Drawing for the job (mm, zero at the part's lowest x, y, z). A direction names the side the tool comes from. Give positions to 0.01 mm unless a question says otherwise; leave off trailing zeros. Order: outer loops, then holes, each group sorted by start corner. A loop starts at its lowest first (then second) coordinate and runs counter-clockwise, first axis right, second up. Notation, with made-up numbers: (35, 0.25) - (54, 0.25) arc R13 cw to (54, 9.25) - close; hole circle Ø1 at (85, 57.5). An arc over 180 degrees is marked (long way). Use a Markdown table: item, result.
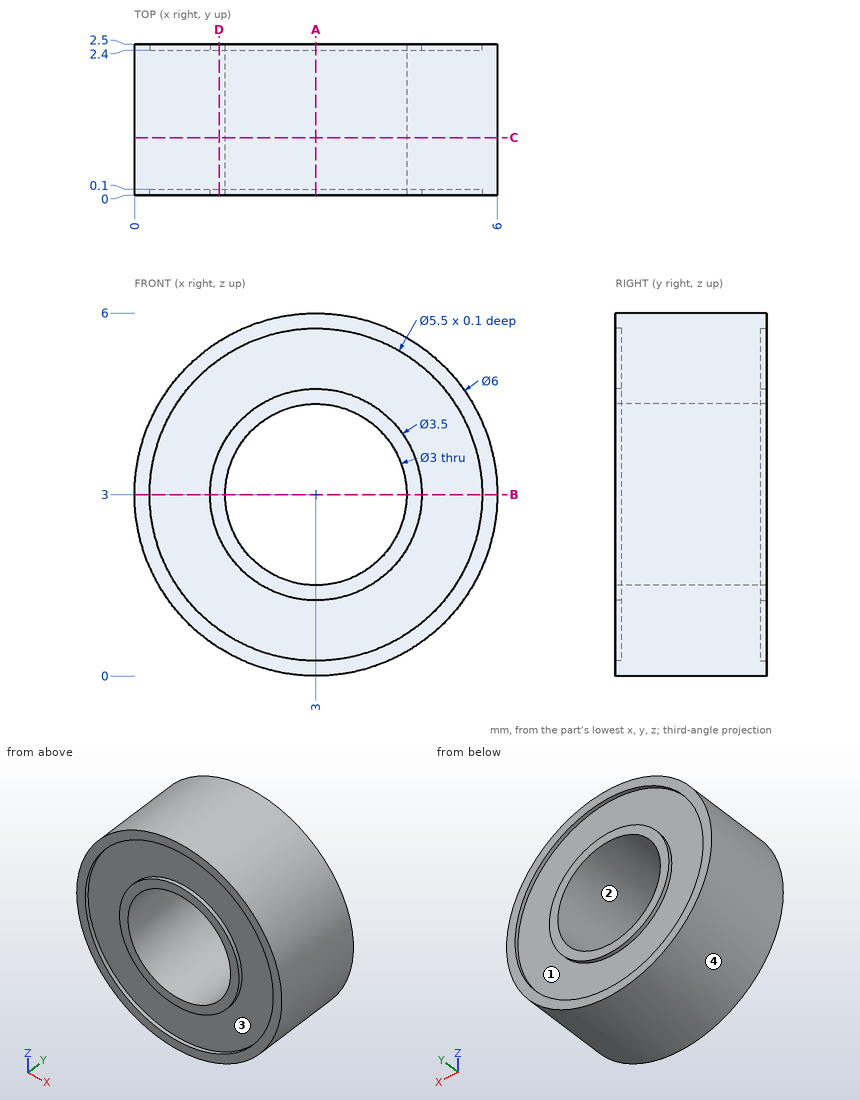
1) Wall check: line 1 (Z direction, x = 3, y = 0.05); line 2 (Z direction, x = 3, y = 0.5); line 3 (X direction, y = 1.35, z = 2.2). Give the ranges that are in metal, low to high. Write a range as from..to.
Computed:
| item | result |
|---|---|
| line 1 | z = 0..0.25, 1.25..1.5, 4.5..4.75, 5.75..6 |
| line 2 | z = 0..1.5, 4.5..6 |
| line 3 | x = 0.11..1.73, 4.27..5.89 |
2) Two-plate mould, pull along Z, no slides. Class the marked faces 3 and 4: +Z half, -Z half, draft (parallel to the pull), parting line (faces both ways), or undercut.
Computed:
| item | result |
|---|---|
| face 3 | undercut |
| face 4 | parting line |
3) Tool access for the marked faces 1 and 2: list every direction of +Z, -Z, +X, -X, +Y, -Y with a clear straight run to the whole face (end or side of a thin tool).
Computed:
| item | result |
|---|---|
| face 1 | +Y |
| face 2 | +Y, -Y |
4) Slice it at C-C (y = 0.95). Write the cut outline in (x, z).
Computed:
| item | result |
|---|---|
| outline | circle Ø6 at (3, 3); hole circle Ø3 at (3, 3) |
5) Slice it at A-A (x = 3). Write the cut outline in (y, z), and give its area (3 significant figures).
Computed:
| item | result |
|---|---|
| outline | (0, 0) - (2.5, 0) - (2.5, 0.25) - (2.4, 0.25) - (2.4, 1.25) - (2.5, 1.25) - (2.5, 1.5) - (0, 1.5) - (0, 1.25) - (0.1, 1.25) - (0.1, 0.25) - (0, 0.25) - close; (0, 4.5) - (2.5, 4.5) - (2.5, 4.75) - (2.4, 4.75) - (2.4, 5.75) - (2.5, 5.75) - (2.5, 6) - (0, 6) - (0, 5.75) - (0.1, 5.75) - (0.1, 4.75) - (0, 4.75) - close |
| area | 7.10 mm² |
6) Pin check, flat tips, straight feed: P1, Ø1.5, axis at y = 0.5, z = 5.5, coming from the +X side; P2, Ø2.5, axis at x = 3, z = 3, coming from the -Y side. Stop position of each tip, or through.
Computed:
| item | result |
|---|---|
| P1 | stops at x = 5.44 |
| P2 | passes through |
7) Slice it at D-D (x = 1.4). Write the cut outline in (y, z).
Computed:
| item | result |
|---|---|
| outline | (0, 0.46) - (2.5, 0.46) - (2.5, 0.76) - (2.4, 0.76) - (2.4, 2.29) - (2.5, 2.29) - (2.5, 3.71) - (2.4, 3.71) - (2.4, 5.24) - (2.5, 5.24) - (2.5, 5.54) - (0, 5.54) - (0, 5.24) - (0.1, 5.24) - (0.1, 3.71) - (0, 3.71) - (0, 2.29) - (0.1, 2.29) - (0.1, 0.76) - (0, 0.76) - close |
8) Slice it at B-B (z = 3). Write the cut outline in (x, y).
Computed:
| item | result |
|---|---|
| outline | (0, 0) - (0.25, 0) - (0.25, 0.1) - (1.25, 0.1) - (1.25, 0) - (1.5, 0) - (1.5, 2.5) - (1.25, 2.5) - (1.25, 2.4) - (0.25, 2.4) - (0.25, 2.5) - (0, 2.5) - close; (4.5, 0) - (4.75, 0) - (4.75, 0.1) - (5.75, 0.1) - (5.75, 0) - (6, 0) - (6, 2.5) - (5.75, 2.5) - (5.75, 2.4) - (4.75, 2.4) - (4.75, 2.5) - (4.5, 2.5) - close |
